Source: three-view drawing plus pictorial views. Frame: mm from the lowest corner of the part. A direction names the side the tool comes from. Give positions to 0.01 mm unless a question says otherwise; leave off trailing zeros. Order: outer loops, then holes, each group sorted by start corner. A loop starts at its lowest first (then second) coordinate and runs counter-clockwise, first axis right, second up.
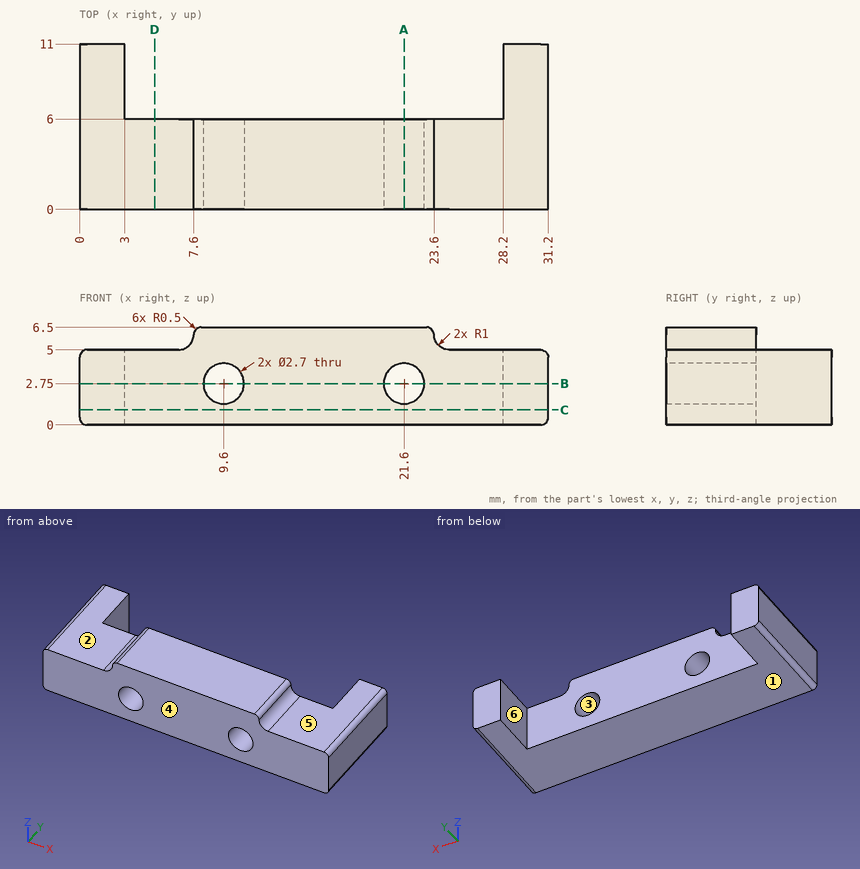
1) Section query B-B on z = 2.75. Output: boundary loops of the cut face in (x, y).
Checks:
outline: (0, 0) - (8.25, 0) - (8.25, 6) - (3, 6) - (3, 11) - (0, 11) - close; (10.95, 0) - (20.25, 0) - (20.25, 6) - (10.95, 6) - close; (22.95, 0) - (31.2, 0) - (31.2, 11) - (28.2, 11) - (28.2, 6) - (22.95, 6) - close
2) Section query C-C on z = 1. Output: boundary loops of the cut face in (x, y), and give its area (3 significant figures).
Checks:
outline: (0, 0) - (31.2, 0) - (31.2, 11) - (28.2, 11) - (28.2, 6) - (3, 6) - (3, 11) - (0, 11) - close
area: 217 mm2
3) Ray query, L1, parallel to X at y = 9, z = 3.25; L2, parallel to Z at x = 21.6, y = 4.6; L3, parallel to Y at x = 13, z = 2.25. Return the intervals inside material, ascending.
Checks:
L1: x = 0 to 3, 28.2 to 31.2
L2: z = 0 to 1.4, 4.1 to 6.5
L3: y = 0 to 6
4) Section query D-D on x = 5. Output: boundary loops of the cut face in (y, z), and give its area (3 significant figures).
Checks:
outline: (0, 0) - (6, 0) - (6, 5) - (0, 5) - close
area: 30.0 mm2
5) Reachability of the marked faces 4, 5 and 6 from +Z, -Z, +X, -X, +Y, -Y: full face, straight path, thin tool, end or side. Return the list, or none.
Checks:
face 4: +Z, -Z, +X, -X, -Y
face 5: +Z, +X, +Y, -Y
face 6: +Z, -Z, +Y
6) Section query A-A on x = 21.6. Output: boundary loops of the cut face in (y, z).
Checks:
outline: (0, 0) - (6, 0) - (6, 1.4) - (0, 1.4) - close; (0, 4.1) - (6, 4.1) - (6, 6.5) - (0, 6.5) - close
7) First-contact query: pin 1 Ø3 at (x, z) = (15.5, 2.5) entering from +Y; pin 2 Ø3 at (x, z) = (21.6, 2.75) entering from -Y; pin 3 Ø5 at (x, y) = (3.5, 3) entering from +Z. Flat tips, straight axial feed; report the tip coordinate or a pass-through.
Checks:
pin 1: stops at y = 6
pin 2: stops at y = 0
pin 3: stops at z = 5
8) Pull-direction query (Z, two-part tool) for the marked faces 1, 2 and 3; classes: +Z half, -Z half, draft (parallel to the pull), parting line (faces both ways), or undercut.
Checks:
face 1: -Z half
face 2: +Z half
face 3: undercut
